Can you work these out from the model? Positions are in its coordinate system, mm. Face numbers are marked on the shaded views. A direction names the side the tool comes from. Round coordinates to 2 decimals unless told otherwise and drop trailing zeros. Write each loop counter-clockwise with the first axis right and the second up, starting at its lowest first coordinate (ties: lowest second). Pieces come first, ordered by that corner, then holes. Notation, with made-up numbers: (46, -36.75) -> (59, -36.75) arc R18 ccw to (59, -17.75) -> close; hole circle Ø5 at (-24, 23). An arc over 180 degrees is marked (long way). Write item = value, one per line. Start each with the question number.
1) I'm going to push flat-ended pins straight in: pin 1 (5.5 mm diameter, centred on x = 0, z = 8.5, fed in from +Y); pin 2 (8 mm diameter, centred on x = 60.5, y = 6, fed in from -Z); pin 3 (1.5 mm diameter, centred on y = 2.5, z = 9.5, fed in from -X); pin 4 (5 mm diameter, centred on x = -6.65, z = 0, fed in from +Y). Where does each tip first touch, or does it pass through?
2) Imagine slicing it at C-C, the plane x = 41. Please give me the cut outline in (y, z).
3) Imagine slicing it at D-D, the plane y = 4.25. Please give me the cut outline in (x, z).
4) For the marked faces 1, 2 and 3, which set-ups out of +Z, -Z, +X, -X, +Y, -Y let a thin tool reach every point of the face, with its end or its side?
5) Thinking about a two-plate mould opening in X: for the marked faces 4, 5 and 6, which applies, +X half, -X half, draft (parallel to the pull), parting line (faces both ways), or undercut?
6) Imagine slicing it at B-B, the plane z = 9.25. Please give me the cut outline in (x, y) (3 decimals).
7) If I drill on line 1 (X direction, y = 5, z = -10); line 2 (X direction, y = -3, z = 13); line 3 (X direction, y = -4, z = 2), over which ranges is the centre line in solid material (lowest first)?
from build123d import *

# Parameters (mm, degrees)
F0_W     = 5.842
F0_H     = 12.7
F0_R     = 3.175
F2_DEPTH = 3.175
F3_R     = 1.524
F4_DEPTH = 7.62
F5_DEPTH = 1.27
F6_DEPTH = 56.134
F7_R     = 1.524
F8_DEPTH = 17.78
F9_DEPTH = 10.414


with BuildPart() as f1:
    # F0 (on Front) → F1 (revolve)
    with BuildSketch(Plane.XZ):
        with Locations((2.921, 6.35)):
            Rectangle(F0_W, F0_H)
        Polygon((5.842, 12.7), (5.842, 0), (66.294, 0), (66.294, 12.7), (56.134, 12.7), (56.134, 10.16), (10.16, 10.16), (10.16, 12.7), align=None)
    revolve(axis=Axis((33.147, 0, 0), (-1, 0, 0)))

    # F0 (on Front) → F2 (join, symmetric)
    with BuildSketch(Plane.XZ):
        with BuildLine():
            Line((-0.9398, 0), (0, 0))
            Line((0, 0), (0, 12.7))
            Line((0, 12.7), (5.842, 12.7))
            Line((5.842, 12.7), (5.842, 15.24))
            Line((5.842, 15.24), (-0.508, 15.24))
            Line((-0.508, 15.24), (-10.8806298187, 3.8475430269))
            ThreePointArc((-10.8806298187, 3.8475430269), (-4.5919612295, 5.3297205562), (-0.9398, 0))
        make_face()
        with BuildLine():
            ThreePointArc((-8.1826630726, -5.5069827884), (-3.1957909266, -4.5493385486), (-0.9398, 0))
            ThreePointArc((-0.9398, 0), (-4.5919612295, 5.3297205562), (-10.8806298187, 3.8475430269))
            ThreePointArc((-10.8806298187, 3.8475430269), (-12.1459778134, -1.5837270034), (-8.1826630726, -5.5069827884))
        make_face()
        with Locations((-6.6548, 0)):
            Circle(F0_R, mode=Mode.SUBTRACT)
        with BuildLine():
            Line((5.842, 0), (0, 0))
            Line((0, 0), (-0.9398, 0))
            ThreePointArc((-0.9398, 0), (-3.1957909266, -4.5493385486), (-8.1826630726, -5.5069827884))
            Line((-8.1826630726, -5.5069827884), (5.842, -9.398))
            Line((5.842, -9.398), (5.842, 0))
        make_face()
        with Locations((2.921, 6.35)):
            Rectangle(F0_W, F0_H)
    extrude(amount=F2_DEPTH, both=True)

    # F3 (on face) → F4 (join)
    with BuildSketch(Plane.YZ.offset(66.294)):
        with BuildLine():
            ThreePointArc((-5.08, 0), (0, -5.08), (5.08, 0))
            ThreePointArc((5.08, 0), (0, 5.08), (-5.08, 0))
        make_face()
        Circle(F3_R, mode=Mode.SUBTRACT)
        with BuildLine():
            ThreePointArc((-5.08, 0), (0, 5.08), (5.08, 0))
            Line((5.08, 0), (5.08, 11.6397422652))
            ThreePointArc((5.08, 11.6397422652), (0, 12.7), (-5.08, 11.6397422652))
            Line((-5.08, 11.6397422652), (-5.08, 0))
        make_face()
        with BuildLine():
            ThreePointArc((-5.08, 11.6397422652), (0, 12.7), (5.08, 11.6397422652))
            Line((5.08, 11.6397422652), (5.08, 15.24))
            Line((5.08, 15.24), (-5.08, 15.24))
            Line((-5.08, 15.24), (-5.08, 11.6397422652))
        make_face()
    extrude(amount=F4_DEPTH)

    # F5 (add): a face of the model
    f5_faces = [f1.faces().sort_by_distance(p)[0] for p in [
        (66.294, 0, 13.7792682875),
    ]]
    extrude(f5_faces, amount=F5_DEPTH)

    # F6 (cut, through all): a face of the model
    f6_faces = [f1.faces().sort_by_distance(p)[0] for p in [
        (66.294, 0, 0),
    ]]
    extrude(f6_faces, amount=-F6_DEPTH, mode=Mode.SUBTRACT)

    # F7 (on face) → F8 (cut)
    with BuildSketch(Plane.XY.offset(15.24)):
        with Locations((2.667, 0)):
            Circle(F7_R)
    extrude(amount=-F8_DEPTH, mode=Mode.SUBTRACT)

    # F7 (on face) → F9 (cut)
    with BuildSketch(Plane.XY.offset(15.24)):
        with Locations((69.469, 0)):
            Circle(F7_R)
    extrude(amount=-F9_DEPTH, mode=Mode.SUBTRACT)


solid = f1.part
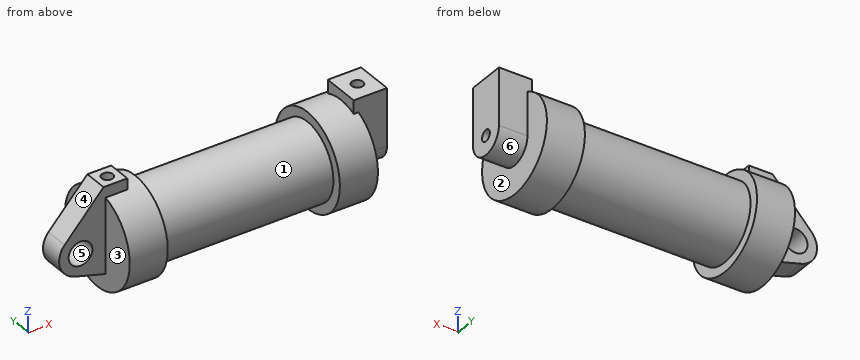
Reported:
q1.pin_1 = 11.32
q1.pin_2 = -12.54
q1.pin_3 = -6.42
q1.pin_4 = through
q2.outline = circle Ø20.32 at (0, 0); hole circle Ø3.05 at (0, 0)
q3.outline = (0, -11.97) -> (10.16, -11.97) -> (10.16, -9.23) -> (56.13, -9.23) -> (56.13, -11.97) -> (66.29, -11.97) -> (66.29, -2.78) -> (73.91, -2.78) -> (73.91, 15.24) -> (65.02, 15.24) -> (65.02, 11.97) -> (56.13, 11.97) -> (56.13, 9.23) -> (10.16, 9.23) -> (10.16, 11.97) -> (0, 11.97) -> close
q4.face_1 = none
q4.face_2 = -Z, +X
q4.face_3 = -Z, -X
q5.face_4 = -X half
q5.face_5 = undercut
q5.face_6 = draft
q6.outline = (-5.962, -3.175) -> (0, -3.175) -> (0, -8.702) -> (10.16, -8.702) -> (10.16, -4.203) -> (56.134, -4.203) -> (56.134, -8.702) -> (66.294, -8.702) -> (66.294, -5.08) -> (73.914, -5.08) -> (73.914, 5.08) -> (66.294, 5.08) -> (66.294, 8.702) -> (56.134, 8.702) -> (56.134, 4.203) -> (10.16, 4.203) -> (10.16, 8.702) -> (0, 8.702) -> (0, 3.175) -> (-5.962, 3.175) -> close; hole circle Ø3.048 at (2.667, 0); hole circle Ø3.048 at (69.469, 0)
q7.line_1 = 0 to 10.16, 56.13 to 66.29
q7.line_2 = -2.55 to 5.84, 65.02 to 73.91
q7.line_3 = 0 to 73.91
